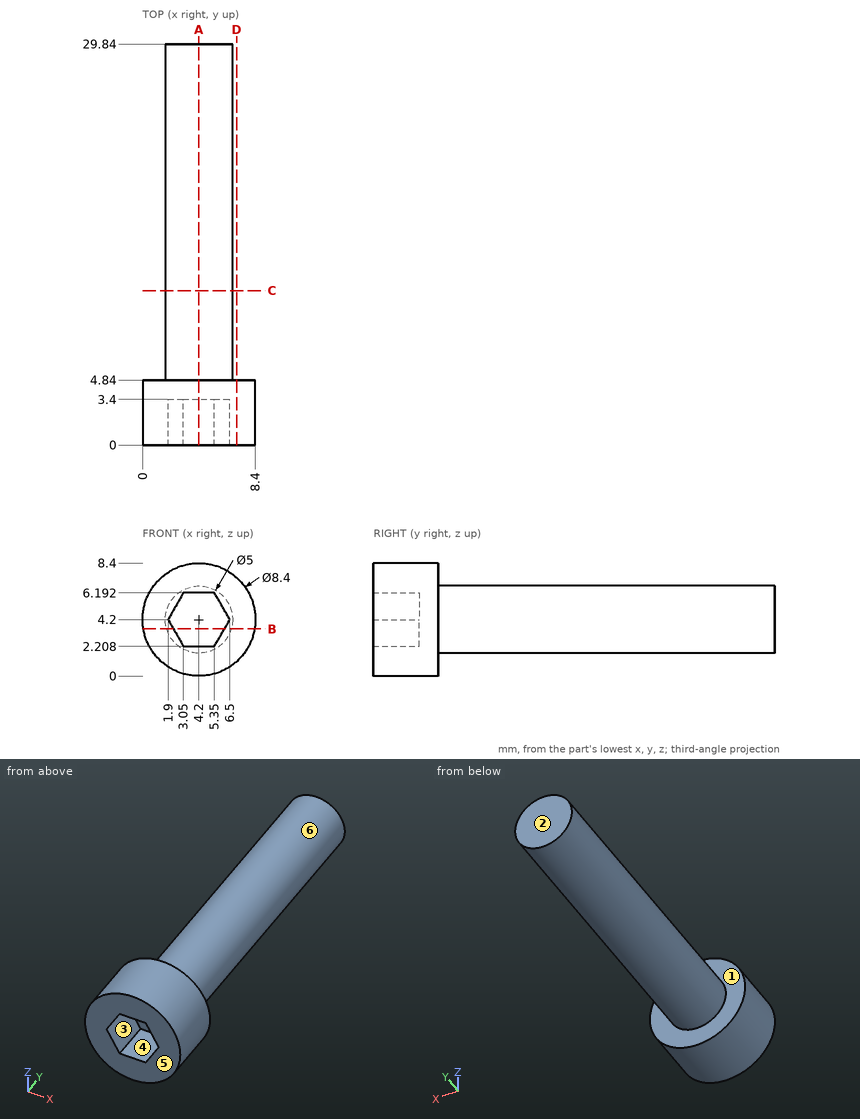
Here's the drawing with two shaded views (mm, measured from the low corner). I have some questions. A direction names the side the tool comes from. Give positions to 0.01 mm unless a question says otherwise; leave off trailing zeros. Loops run counter-clockwise (first coordinate to the right, second up) from the corner with the lowest first, then second, coordinate; pieces in that order, holes last. Notation, with made-up numbers: M 81.25,83.5 L 96.25,83.5 A31 cw 96.25,117.5 Z; hole C -36,-30 d4. An arc over 180 degrees is marked long. Use one line per item in the form item = value. Start each with the question number.
(1) I want a section at C-C, the plane y = 11.5. Write out the boundary of the cut face in (x, z), and give its area (3 significant figures).
(2) I want a section at D-D, the plane x = 7. Write out the boundary of the cut face in (y, z).
(3) Please list where these lines run through material, in increasing order: line 1 (Y direction, x = 7, z = 3.25); line 2 (Y direction, x = 3.5, z = 3); line 3 (X direction, y = 6, z = 6) (1 decimal).
(4) I'm going to push flat-ended pins straight in: P1, Ø1.5, axis at x = 7, y = 11, coming from the +Z side; P2, Ø3, axis at y = 10.5, z = 1, coming from the -X side; P3, Ø4, axis at y = 20.5, z = 6, coming from the -X side. Where does each tip first touch, or does it pass through?
(5) On a 3-axis mill with a long thin cutter (end or side, diameter ignored), from which of +Z, -Z, +X, -X, +Y, -Y can I reach the whole of each face in a straight line? I mean the marked faces 1 and 2. Say none if no direction works.
(6) I want a section at B-B, the plane z = 3.5. Write out the boundary of the cut face in (x, y).
(7) I want a section at A-A, the plane x = 4.2. Write out the boundary of the cut face in (y, z).
(8) Thinking about a two-plate mould opening in Z: for the marked faces 3, 4, 5 and 6, which applies, released by +Z, released by -Z, zero draft, split by the parting line, or undercut?
Worked out:
q1.outline = C 4.2,4.2 d5
q1.area = 19.6 mm²
q2.outline = M 0,1.07 L 4.84,1.07 L 4.84,7.33 L 0,7.33 Z
q3.line_1 = 0 to 4.84
q3.line_2 = 3.4 to 29.84
q3.line_3 = 2.5 to 5.9
q4.P1 = 5.63
q4.P2 = 2.37
q4.P3 = 1.7
q5.face_1 = +Y
q5.face_2 = +Z, -Z, +X, -X, +Y
q6.outline = M 0.06,0 L 2.3,0 L 2.3,3.4 L 6.1,3.4 L 6.1,0 L 8.34,0 L 8.34,4.84 L 6.6,4.84 L 6.6,29.84 L 1.8,29.84 L 1.8,4.84 L 0.06,4.84 Z
q7.outline = M 0,0 L 4.84,0 L 4.84,1.7 L 29.84,1.7 L 29.84,6.7 L 4.84,6.7 L 4.84,8.4 L 0,8.4 L 0,6.19 L 3.4,6.19 L 3.4,2.21 L 0,2.21 Z
q8.face_3 = undercut
q8.face_4 = undercut
q8.face_5 = zero draft
q8.face_6 = split by the parting line
